Source: three-view drawing plus pictorial views. Frame: mm from the lowest corner of the part. A direction names the side the tool comes from. Give positions to 0.01 mm unless a question says otherwise; leave off trailing zeros. Loops run counter-clockwise (first coordinate to the right, second up) from the corner with the lowest first, then second, coordinate; pieces in that order, holes last.
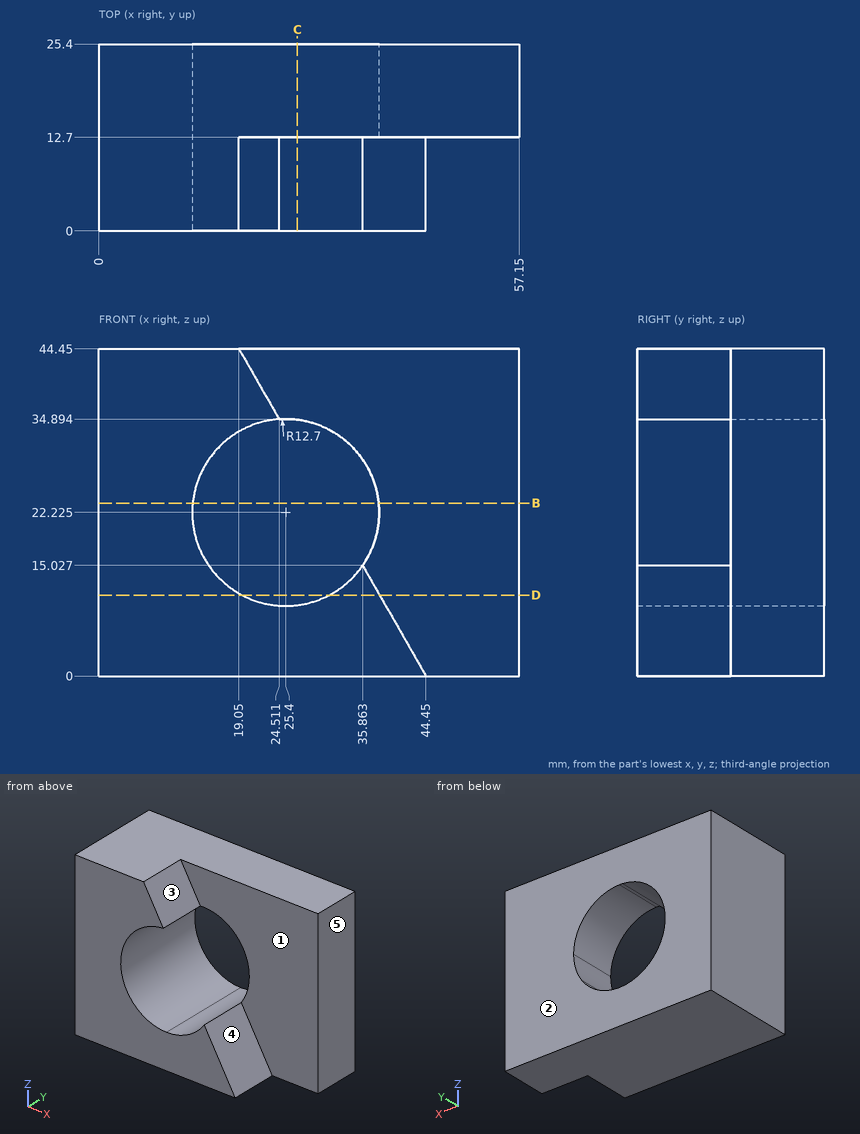
1) Ray query, probe 1 along X at (y, z) = (8.5, 22); probe 2 along Y at (x, z) = (47, 15); probe 3 along Z at (x, y) = (15.5, 2.75). Return the intervals inside material, ascending.
Checks:
probe 1: x = 0 to 12.7
probe 2: y = 12.7 to 25.4
probe 3: z = 0 to 14.27, 30.18 to 44.45
2) Cut plane C-C (x = 27). Return loops of the section in (y, z), and give its area (3 significant figures).
Checks:
outline: (0, 0) - (25.4, 0) - (25.4, 9.63) - (0, 9.63) - close; (12.7, 34.82) - (25.4, 34.82) - (25.4, 44.45) - (12.7, 44.45) - close
area: 367 mm2
3) Contact query for flat-ended pins moving along their axis: P1, Ø8, axis at x = 35, z = 12, coming from the -Y side; P2, Ø10, axis at x = 42, z = 34.5, coming from the -Y side; P3, Ø6, axis at y = 5.5, z = 12, coming from the +X side. Output: stop coordinate, or through.
Checks:
P1: stops at y = 0
P2: stops at y = 12.7
P3: stops at x = 39.31
4) Cut plane B-B (z = 23.5). Return loops of the section in (x, y).
Checks:
outline: (0, 0) - (12.76, 0) - (12.76, 25.4) - (0, 25.4) - close; (38.04, 12.7) - (57.15, 12.7) - (57.15, 25.4) - (38.04, 25.4) - close
5) Cut plane D-D (z = 11). Return loops of the section in (x, y), and give its area (3 significant figures).
Checks:
outline: (0, 0) - (19.46, 0) - (19.46, 25.4) - (0, 25.4) - close; (31.34, 0) - (38.16, 0) - (38.16, 12.7) - (57.15, 12.7) - (57.15, 25.4) - (31.34, 25.4) - close
area: 909 mm2
6) Pull-direction query (Y, two-part tool) for the marked faces 1, 2 and 3; classes: released by +Y, released by -Y, zero draft, split by the parting line, or undercut.
Checks:
face 1: released by -Y
face 2: released by +Y
face 3: zero draft
7) Reachability of the marked faces 4 and 5 from +Z, -Z, +X, -X, +Y, -Y: full face, straight path, thin tool, end or side. Return the list, or none.
Checks:
face 4: +Z, +X, -Y
face 5: +Z, -Z, +X, +Y, -Y
